Build history of the part. All positions in model axes, mm. Face numbers are marked on the shaded views. Give positions to 0.01 mm unless a question says otherwise; leave off trailing zeros. Loops run counter-clockwise (first coordinate to the right, second up) from the corner with the lowest first, then second, coordinate; pieces in that order, holes last. Notation, with made-up numbers: (-4, -33.75) -> (27, -33.75) arc R29 ccw to (27, -10.75) -> close; hole circle Ø1 at (63.5, 22.25). An arc over 180 degrees is marked (long way). Answer as a JSON object with one key per item and string values. Group by question number.
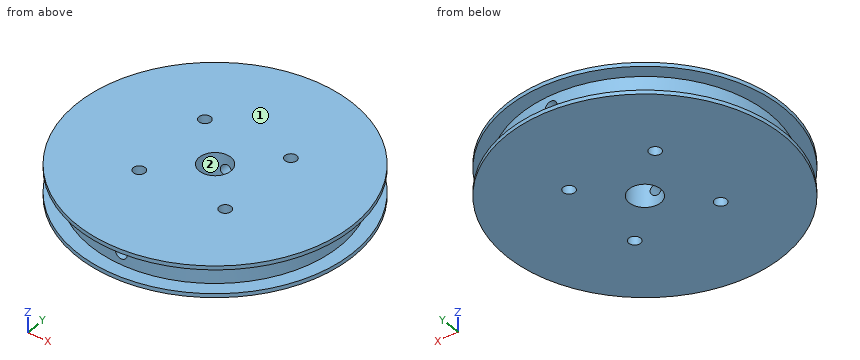
from build123d import *

# Parameters (mm, degrees)
SKETCH1_R                                       = 35
PULLEY_BOSS_EXTRUDE1_DEPTH                      = 8
SKETCH2_W                                       = 3.5
SKETCH2_H                                       = 6
SKETCH3_R                                       = 4
SHAFT_CUT_EXTRUDE1_DEPTH                        = 8
SPRINT_HOLE_CUT_EXTRUDE2_REACH                  = 52.14
SPRINT_HOLE_CUT_EXTRUDE2_END_RADIUS             = 31.5
SKETCH4_R                                       = 1.5
SPRINT_HOLE_CUT_EXTRUDE2_DIRECTION_2_REACH      = 52.14
SPRINT_HOLE_CUT_EXTRUDE2_DIRECTION_2_END_RADIUS = 31.5
SKETCH5_R                                       = 1.5
ARM_DISTANS_MOUNTING_HOLES_CUT_EXTRUDE1_DEPTH   = 8


with BuildPart() as part:
    # Sketch1 → Pulley Boss-Extrude1 (new body)
    with BuildSketch(Plane.XY):
        Circle(SKETCH1_R)
    extrude(amount=PULLEY_BOSS_EXTRUDE1_DEPTH)

    # Sketch2 → Belt Cut-Revolve3 (revolve, cut)
    with BuildSketch(Plane(origin=(0, 0, 0), x_dir=(1, 0, 0), z_dir=(0, 1, 0)), mode=Mode.PRIVATE) as belt_cut_revolve3_sk:
        with Locations((33.25, -4)):
            Rectangle(SKETCH2_W, SKETCH2_H)
    revolve(belt_cut_revolve3_sk.sketch.rotate(Axis((0, 0, -14.62158436), (0, 0, 1)), 180), axis=Axis((0, 0, -14.62158436), (0, 0, 1)), mode=Mode.SUBTRACT)

    # Sketch3 → Shaft Cut-Extrude1 (cut)
    with BuildSketch(Plane.XY):
        with Locations(Location((0, 0, 0), (0, 0, 180))):
            Circle(SKETCH3_R)
    extrude(amount=SHAFT_CUT_EXTRUDE1_DEPTH, mode=Mode.SUBTRACT)

    # Sprint Hole Cut-Extrude2: up to this cylinder (the profile starts inside it)
    sprint_hole_cut_extrude2_end = Plane(origin=(0, 0, 4), z_dir=(0, 0, -1)) * Cylinder(SPRINT_HOLE_CUT_EXTRUDE2_END_RADIUS, 168.28, mode=Mode.PRIVATE)
    # Sketch4 → Sprint Hole Cut-Extrude2 (cut, up to the surface)
    with BuildSketch(Plane(origin=(0, 0, 0), x_dir=(1, 0, 0), z_dir=(0, 1, 0)), mode=Mode.PRIVATE) as sprint_hole_cut_extrude2_sk1:
        with Locations(Location((0, -4, 0), (0, 0, 270))):
            Circle(SKETCH4_R)
    sprint_hole_cut_extrude2_tool1 = extrude(sprint_hole_cut_extrude2_sk1.sketch, amount=-SPRINT_HOLE_CUT_EXTRUDE2_REACH, mode=Mode.PRIVATE) & sprint_hole_cut_extrude2_end
    add(sprint_hole_cut_extrude2_tool1.solids().sort_by_distance((0, 0, 4))[0], mode=Mode.SUBTRACT)

    # Sprint Hole Cut-Extrude2 direction 2: up to this cylinder (the profile starts inside it)
    sprint_hole_cut_extrude2_direction_2_end = Plane(origin=(0, 0, 4), z_dir=(0, 0, -1)) * Cylinder(SPRINT_HOLE_CUT_EXTRUDE2_DIRECTION_2_END_RADIUS, 168.28, mode=Mode.PRIVATE)
    # Sketch4 → Sprint Hole Cut-Extrude2 direction 2 (cut, up to the surface)
    with BuildSketch(Plane(origin=(0, 0, 0), x_dir=(1, 0, 0), z_dir=(0, 1, 0)), mode=Mode.PRIVATE) as sprint_hole_cut_extrude2_direction_2_sk1:
        with Locations(Location((0, -4, 0), (0, 0, 270))):
            Circle(SKETCH4_R)
    sprint_hole_cut_extrude2_direction_2_tool1 = extrude(sprint_hole_cut_extrude2_direction_2_sk1.sketch, amount=SPRINT_HOLE_CUT_EXTRUDE2_DIRECTION_2_REACH, mode=Mode.PRIVATE) & sprint_hole_cut_extrude2_direction_2_end
    add(sprint_hole_cut_extrude2_direction_2_tool1.solids().sort_by_distance((0, 0, 4))[0], mode=Mode.SUBTRACT)

    # Sketch5 → Arm Distans Mounting Holes Cut-Extrude1 (cut)
    with BuildSketch(Plane.XY.offset(8)):
        with Locations((11, 11)):
            Circle(SKETCH5_R)
        with Locations((-11, 11)):
            Circle(SKETCH5_R)
        with Locations((-11, -11)):
            Circle(SKETCH5_R)
        with Locations((11, -11)):
            Circle(SKETCH5_R)
    extrude(amount=-ARM_DISTANS_MOUNTING_HOLES_CUT_EXTRUDE1_DEPTH, mode=Mode.SUBTRACT)


solid = part.part
(1) Pull direction Y, two halves, no side cores. Call the marked faces 1 and 2: pulls with the +Y half, pulls with the -Y half, needs draft (parallel to the pull), parting line crosses it, or undercut.
(2) Probe line 1 along Z through (x, y) = (-24, -21); line 2 along Z through (x, y) = (0, 17); line 3 along X through (y, z) = (-19.5, 4). List the from-to ranges inside material, lowest first. Write a range as [from, to].
(3) Saw through at A-A on y = 0. List the corners of the cut face in (x, z), plus the area to 3 significant figures.
(4) Pin check, flat tips, straight feed: pin 1 (1.5 mm diameter, centred on x = -27, y = -7.5, fed in from -Z); pin 2 (3 mm diameter, centred on x = -5, z = 5, fed in from -Y); pin 3 (4 mm diameter, centred on y = -13.5, z = 6, fed in from -X). Stop position of each tip, or through.
(5) Saw through at D-D on y = 11. List the corners of the cut face in (x, z), plus the area to 3 significant figures.
(6) Saw through at C-C on x = -11.5. List the corners of the cut face in (y, z).
(7) Saw through at B-B on z = 3.5. List the corners of the cut face in (x, y), plus the area to 3 significant figures.
Calculated:
{
 "1": {"face 1": "needs draft", "face 2": "undercut"},
 "2": {"line 1": "z = [0, 1], [7, 8]", "line 2": "z = [0, 2.5], [5.5, 8]", "line 3": "x = [-24.74, -1.5], [1.5, 24.74]"},
 "3": {"outline": "(-35, 0) -> (-4, 0) -> (-4, 8) -> (-35, 8) -> (-35, 7) -> (-31.5, 7) -> (-31.5, 1) -> (-35, 1) -> close; (4, 0) -> (35, 0) -> (35, 1) -> (31.5, 1) -> (31.5, 7) -> (35, 7) -> (35, 8) -> (4, 8) -> close", "area": "454 mm^2"},
 "4": {"pin 1": "stops at z = 0", "pin 2": "stops at y = -31.3", "pin 3": "stops at x = -32.96"},
 "5": {"outline": "(-33.23, 0) -> (-12.5, 0) -> (-12.5, 8) -> (-33.23, 8) -> (-33.23, 7) -> (-29.52, 7) -> (-29.52, 1) -> (-33.23, 1) -> close; (-9.5, 0) -> (9.5, 0) -> (9.5, 8) -> (-9.5, 8) -> close; (12.5, 0) -> (33.23, 0) -> (33.23, 1) -> (29.52, 1) -> (29.52, 7) -> (33.23, 7) -> (33.23, 8) -> (12.5, 8) -> close; hole circle Ø3 at (0, 4)", "area": "432 mm^2"},
 "6": {"outline": "(-33.06, 0) -> (-12.41, 0) -> (-12.41, 8) -> (-33.06, 8) -> (-33.06, 7) -> (-29.33, 7) -> (-29.33, 1) -> (-33.06, 1) -> close; (-9.59, 0) -> (9.59, 0) -> (9.59, 8) -> (-9.59, 8) -> close; (12.41, 0) -> (33.06, 0) -> (33.06, 1) -> (29.33, 1) -> (29.33, 7) -> (33.06, 7) -> (33.06, 8) -> (12.41, 8) -> close"},
 "7": {"outline": "(-1.41, -31.47) -> (-1.41, -3.74) arc R4 cw to (-1.41, 3.74) -> (-1.41, 31.47) arc R31.5 ccw to start; (1.41, -31.47) arc R31.5 ccw to (1.41, 31.47) -> (1.41, 3.74) arc R4 cw to (1.41, -3.74) -> close; hole circle Ø3 at (-11, -11); hole circle Ø3 at (-11, 11); hole circle Ø3 at (11, -11); hole circle Ø3 at (11, 11)", "area": "2,880 mm^2"}
}
